from build123d import *

# Parameters (mm, degrees)
SKETCH_1_R               = 7.5
SKETCH_1_R_2             = 2.05
EXTRUDE_1_DEPTH          = 15
EXTRUDE_2_DEPTH          = 22.5
SKETCH_3_R               = 22.6
CUT_EXTRUDE_1_DEPTH      = 125
SKETCH_5_W               = 80
SKETCH_5_H               = 15
CUT_EXTRUDE_2_DEPTH      = 15
CUT_EXTRUDE_3_DEPTH      = 131.008833765
CUT_EXTRUDE_3_DEPTH_BACK = 131.008833765
SKETCH_6_R               = 1.95
CUT_EXTRUDE_4_DEPTH      = 131.008833765
CUT_EXTRUDE_4_DEPTH_BACK = 131.008833765
SKETCH_10_R              = 1.95
CUT_EXTRUDE_5_DEPTH      = 131.008833765
CUT_EXTRUDE_5_DEPTH_BACK = 131.008833765
SKETCH_11_R              = 2.05
CUT_EXTRUDE_6_DEPTH      = 3.1
SKETCH_16_W              = 100
SKETCH_16_H              = 15.085035438
CUT_EXTRUDE_7_DEPTH      = 5
CHAMFER_1_SIZE           = 2
SKETCH_17_R              = 3.5
CUT_EXTRUDE_8_DEPTH      = 4
SKETCH_19_W              = 12
SKETCH_19_H              = 8
CUT_EXTRUDE_10_DEPTH     = 5
SKETCH_20_W              = 30
SKETCH_20_H              = 18.196576595
CUT_EXTRUDE_12_DEPTH     = 1.5
SKETCH_21_R              = 1.925
CUT_EXTRUDE_13_DEPTH     = 5


with BuildPart() as part:
    # 스케치1 → 보스-돌출1 (new, symmetric)
    # profile 1 of 2: a face of its own
    with BuildSketch(Plane(origin=(0, 0, 0), x_dir=(0, 0, -1), z_dir=(1, 0, 0))):
        with BuildLine():
            ThreePointArc((7.5, 0), (5.303300859, -5.303300859), (0, -7.5))
            Line((0, -7.5), (37.938480529, -7.5))
            Line((37.938480529, -7.5), (36.613399157, 7.5))
            Line((36.613399157, 7.5), (0, 7.5))
            ThreePointArc((0, 7.5), (5.303300859, 5.303300859), (7.5, 0))
        make_face()
    # profile 2 of 2: a face of its own
    with BuildSketch(Plane(origin=(0, 0, 0), x_dir=(0, 0, -1), z_dir=(1, 0, 0))):
        Circle(SKETCH_1_R)
        Circle(SKETCH_1_R_2, mode=Mode.SUBTRACT)
    extrude(amount=EXTRUDE_1_DEPTH, both=True)

    # 스케치2 → 보스-돌출2 (add, symmetric)
    with BuildSketch(Plane(origin=(0, 0, 0), x_dir=(0, 0, -1), z_dir=(1, 0, 0))):
        Polygon((15.1, 3.389248282), (15.1, 14), (127.279404685, 14), (120, -6), (19.447603562, -6), align=None)
    extrude(amount=EXTRUDE_2_DEPTH, both=True)

    # 스케치3 → 컷-돌출1 (cut)
    with BuildSketch(Plane.XY.offset(-150)):
        with Locations((0, 30)):
            Circle(SKETCH_3_R)
    extrude(amount=CUT_EXTRUDE_1_DEPTH, mode=Mode.SUBTRACT)

    # 스케치5 → 컷-돌출2 (cut)
    with BuildSketch(Plane(origin=(22.5, 0, 0), x_dir=(0, 0, -1), z_dir=(1, 0, 0))):
        with Locations((100, -3.5)):
            Rectangle(SKETCH_5_W, SKETCH_5_H)
    cut_extrude_2 = extrude(amount=-CUT_EXTRUDE_2_DEPTH, mode=Mode.SUBTRACT)

    # 대칭 복사1: 컷-돌출2 across plane
    add(cut_extrude_2.mirror(Plane(origin=(0, 0, 0), x_dir=(0, 0, 1), z_dir=(1, 0, 0))), mode=Mode.SUBTRACT)

    # 스케치6 → 컷-돌출3 (cut, two sides: drawn at the far end of the back side and taken through both)
    with BuildSketch(Plane(origin=(0, 0, 0), x_dir=(0, 0, -1), z_dir=(1, 0, 0)).offset(-CUT_EXTRUDE_3_DEPTH_BACK)):
        with Locations((70, -1)):
            Circle(SKETCH_6_R)
        with Locations((110, -1)):
            Circle(SKETCH_6_R)
    extrude(amount=CUT_EXTRUDE_3_DEPTH + CUT_EXTRUDE_3_DEPTH_BACK, mode=Mode.SUBTRACT)

    # 스케치10 → 컷-돌출4 (cut, two sides: drawn at the far end of the back side and taken through both)
    with BuildSketch(Plane(origin=(0, 0, 0), x_dir=(0, 0, -1), z_dir=(1, 0, 0)).offset(-CUT_EXTRUDE_4_DEPTH_BACK)):
        with Locations((27, 0)):
            Circle(SKETCH_10_R)
    extrude(amount=CUT_EXTRUDE_4_DEPTH + CUT_EXTRUDE_4_DEPTH_BACK, mode=Mode.SUBTRACT)

    # 스케치11 → 컷-돌출5 (cut, two sides: drawn at the far end of the back side and taken through both)
    with BuildSketch(Plane(origin=(0, 0, 0), x_dir=(0, 0, -1), z_dir=(1, 0, 0)).offset(-CUT_EXTRUDE_5_DEPTH_BACK)):
        with Locations((35.850364983, -1)):
            Circle(SKETCH_11_R)
    extrude(amount=CUT_EXTRUDE_5_DEPTH + CUT_EXTRUDE_5_DEPTH_BACK, mode=Mode.SUBTRACT)

    # 스케치12 → 컷-돌출6 (cut, symmetric)
    with BuildSketch(Plane(origin=(0, 0, 0), x_dir=(0, 0, -1), z_dir=(1, 0, 0))):
        with BuildLine():
            Line((30.150364983, -1), (30.150364983, 12.943670284))
            ThreePointArc((30.150364983, 12.943670284), (35.850364983, 18.643670284), (41.550364983, 12.943670284))
            Line((41.550364983, 12.943670284), (41.550364983, -1))
            ThreePointArc((41.550364983, -1), (35.850364983, -6.7), (30.150364983, -1))
        make_face()
    extrude(amount=CUT_EXTRUDE_6_DEPTH, both=True, mode=Mode.SUBTRACT)

    # 스케치16 → 컷-돌출7 (cut, symmetric)
    with BuildSketch(Plane(origin=(0, 0, 0), x_dir=(0, 0, -1), z_dir=(1, 0, 0))):
        with Locations((70, -12.542517719)):
            Rectangle(SKETCH_16_W, SKETCH_16_H)
    extrude(amount=CUT_EXTRUDE_7_DEPTH, both=True, mode=Mode.SUBTRACT)

    # 모따기1
    chamfer_1_edges = [part.edges().sort_by_distance(p)[0] for p in [
        (-22.5, 14, -71.189702343),
        (22.5, 14, -71.189702343),
    ]]
    chamfer(chamfer_1_edges, length=CHAMFER_1_SIZE)

    # 스케치17 → 컷-돌출8 (cut)
    with BuildSketch(Plane(origin=(22.5, 0, 0), x_dir=(0, 0, -1), z_dir=(1, 0, 0))):
        with Locations((35.850364983, -1)):
            Circle(SKETCH_17_R)
    extrude(amount=-CUT_EXTRUDE_8_DEPTH, mode=Mode.SUBTRACT)

    # 스케치19 → 컷-돌출10 (cut)
    with BuildSketch(Plane(origin=(0, 14, 0), x_dir=(1, 0, 0), z_dir=(0, 1, 0))):
        with Locations((0, 19.1)):
            Rectangle(SKETCH_19_W, SKETCH_19_H)
    extrude(amount=-CUT_EXTRUDE_10_DEPTH, mode=Mode.SUBTRACT)

    # 스케치20 → 컷-돌출12 (cut)
    with BuildSketch(Plane.XZ.offset(6)):
        with Locations((0, -29.098288298)):
            Rectangle(SKETCH_20_W, SKETCH_20_H)
    extrude(amount=CUT_EXTRUDE_12_DEPTH, mode=Mode.SUBTRACT)

    # 스케치21 → 컷-돌출13 (cut)
    with BuildSketch(Plane.XZ.offset(6)):
        with Locations(Location((12, -42, 0), (0, 0, 270))):
            Circle(SKETCH_21_R)
        with Locations(Location((-12, -42, 0), (0, 0, 90))):
            Circle(SKETCH_21_R)
    extrude(amount=-CUT_EXTRUDE_13_DEPTH, mode=Mode.SUBTRACT)


solid = part.part
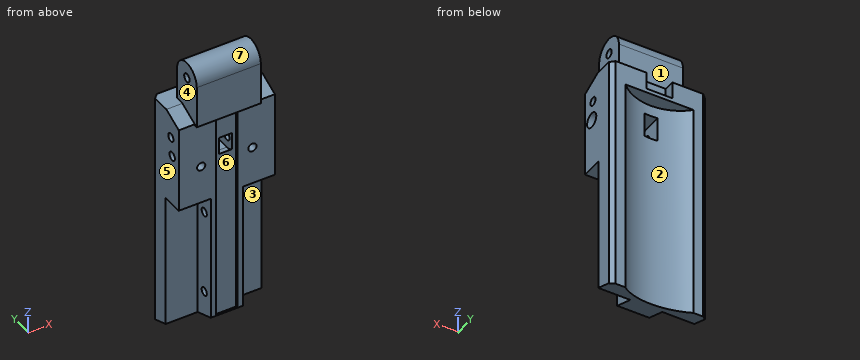
The listing builds one solid part. Answer for the finished solid, in the listing's coordinates (mm). Face numbers are marked on the shaded views. A direction names the side the tool comes from. Coordinates: 2 decimals unless noted, no trailing zeros. Order: outer loops, then holes, each group sorted by start corner. A loop starts at its lowest first (then second) coordinate and runs counter-clockwise, first axis right, second up.
Q1. A cutting plane is placed at C-C, the plane z = -86.5. Write down the section's boundary in (x, y), and give its area (3 significant figures).
Q2. Given P1, Ø0.5, axis at y = -5.5, z = -73.5, coming from the -X side; P2, Ø14, axis at x = 11, z = -77.5, coming from the -Y side; P3, Ø1, axis at x = 17, y = 0.5, coming from the -Z side; P4, Ø3.5, axis at y = -1, z = -35.85, coming from the +X side, each flat-ended and moving along its own axis, determine where each tip first touches the part or whether it passes through.
Q3. For a pull along Z with two mould halves and no side action, classify the marked faces 5, 6 and 7 as pulls with the +Z half, pulls with the -Z half, needs draft (parallel to the pull), parting line crosses it, or undercut.
Q4. Which of the six approach directions +Z, -Z, +X, -X, +Y, -Y give full straight-line access (tool end or side, diameter ignored) to the marked faces 1, 2, 3 and 4?
Q5. A cutting plane is placed at B-B, the plane z = -27. Write down the section's boundary in (x, y).
Q6. A cutting plane is placed at D-D, the plane x = 12. Write down the section's boundary in (y, z) (3 decimals).
Q7. Consider line 1 (X direction, y = -2.4, z = -42) (3 decimals); line 2 (Z direction, x = 14.75, y = -1); line 3 (Y direction, x = 2, z = 0). Determine where each line is inside the solid, lowest interval first.
Q8. A cutting plane is placed at A-A, the plane x = -1. Write down the section's boundary in (y, z).
Answers follow:
1. outline: (-22.5, 4) - (-7.5, 4) - (-7.5, -6) - (-5, -6) - (-5, -5) - (5, -5) - (5, -6) - (7.5, -6) - (7.5, 4) - (22.5, 4) - (22.5, 12) - (20.5, 14) - (15.96, 14) arc R22.6 cw to (-15.96, 14) - (-20.5, 14) - (-22.5, 12) - close
1. area: 441 mm2
2. P1: stops at x = -7.5
2. P2: stops at y = -6
2. P3: stops at z = -60
2. P4: passes through
3. face 5: needs draft
3. face 6: undercut
3. face 7: pulls with the +Z half
4. face 1: +Z, +X, -X, +Y
4. face 2: -Z, +Y
4. face 3: -Z, +X, -Y
4. face 4: +Z, -X, -Y
5. outline: (-22.5, -6) - (-5, -6) - (-5, -5) - (5, -5) - (5, -6) - (22.5, -6) - (22.5, -1.95) - (-22.5, -1.95) - close; (-22.5, 1.95) - (22.5, 1.95) - (22.5, 12) - (20.5, 14) - (15.96, 14) arc R22.6 cw to (-15.96, 14) - (-20.5, 14) - (-22.5, 12) - close
6. outline: (-7.5, -20) - (-6, -20) - (-6, -40.075) - (-1, -40.075) - (-1, -43.925) - (-6, -43.925) - (-6, -60) - (4, -60) - (4, -123.64) - (10.849, -126.133) - (10.849, -25) - (14, -25) - (14, -15.1) - (7.5, -15.1) - (7.5, 0) arc R7.5 ccw to (-7.5, 0) - close; hole circle Ø4.1 at (-1, -35.85); hole circle Ø4.1 at (0, 0); hole circle Ø3.9 at (0, -27)
7. line 1: x = -22.5 to -13.925, -10.075 to 10.075, 13.925 to 22.5
7. line 2: z = -60 to -37.9, -33.8 to -28.67, -25.33 to -1.79, 1.79 to 7.43
7. line 3: y = -7.5 to -2.05, 2.05 to 7.5
8. outline: (-7.5, -20) - (-5, -20) - (-5, -31.79) arc R5.7 cw to (-1, -30.15) - (7.42, -30.15) - (7.42, -25) - (14, -25) - (14, -23.1) - (9, -23.1) - (9, -15.1) - (7.5, -15.1) - (7.5, 0) arc R7.5 ccw to (-7.5, 0) - close; (-6, -120) - (7.42, -124.89) - (7.42, -41.55) - (-1, -41.55) arc R5.7 cw to (-5, -39.91) - (-5, -120) - close; hole circle Ø3.9 at (-1, -110); hole circle Ø3.9 at (-1, -70); hole circle Ø4.1 at (0, 0); hole circle Ø3.9 at (0, -27)
